Can you work these out from the model? Positions are in its coordinate system, mm. Face numbers are marked on the shaded views. A direction names the side the tool comes from. Coordinates: 2 decimals unless noted, no trailing zeros. Loops run counter-clockwise (first coordinate to the right, second up) from the corner with the lowest first, then second, coordinate; pieces in that order, holes last. Notation, with made-up numbers: M 3.5,22.5 L 27.5,22.5 A21 ccw 27.5,42.5 Z; hole C 34.25,20 d1. An arc over 180 degrees is marked long. Return JSON: item names as keys, results as strings. Group by question number.
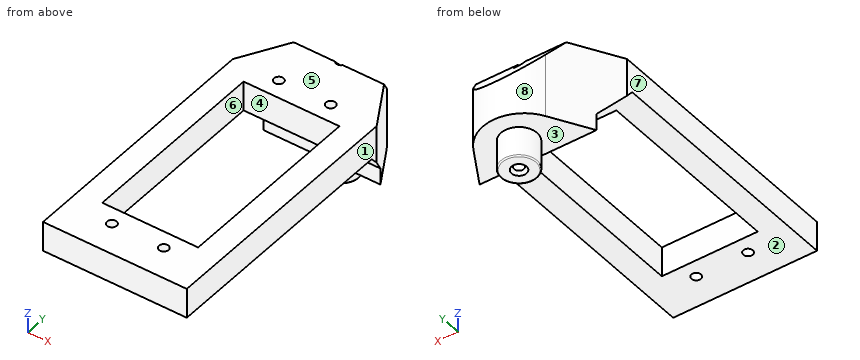
```python
from build123d import *

# Parameters (mm, degrees)
F0_R           = 1.016
F0_W           = 20.32
F0_H           = 40.64
F2_DEPTH       = 17.526
F3_START       = -25.4
F3_DEPTH       = 40.641
F4_R           = 3.81
F5_DEPTH       = 6.35
F7_D           = 2.032
F7_CSINK_D     = 3.175
F7_CSINK_ANGLE = 82
F8_R           = 0.254


with BuildPart() as f2:
    # F0 (on Top) → F2 (new body, through all)
    with BuildSketch(Plane.XY):
        with BuildLine():
            Line((-15.24, -40.64), (15.24, -40.64))
            Line((15.24, -40.64), (15.24, 13.97))
            Line((15.24, 13.97), (7.62, 27.1682271537))
            ThreePointArc((7.62, 27.1682271537), (0, 31.6135833353), (-7.62, 27.1682271537))
            Line((-7.62, 27.1682271537), (-15.24, 13.97))
            Line((-15.24, 13.97), (-15.24, -40.64))
        make_face()
        with Locations((-5.4991, -34.036)):
            Circle(F0_R, mode=Mode.SUBTRACT)
        with Locations((5.4991, -34.036)):
            Circle(F0_R, mode=Mode.SUBTRACT)
        with Locations((0, -10.16)):
            Rectangle(F0_W, F0_H, mode=Mode.SUBTRACT)
        with Locations((-5.4991, 13.97)):
            Circle(F0_R, mode=Mode.SUBTRACT)
        with Locations((5.4991, 13.97)):
            Circle(F0_R, mode=Mode.SUBTRACT)
    extrude(amount=F2_DEPTH)

    # F1 (on Right) → F3 (intersect)
    with BuildSketch(Plane.YZ.offset(F3_START)):
        Polygon((18.9135833353, 3.556), (18.9135833353, 0), (31.6135833353, 0), (31.6135833353, 8.1784219752), (23.7700340623, 17.526), (-40.64, 17.526), (-40.64, 11.176), (12.5196441457, 11.176), align=None)
    extrude(amount=F3_DEPTH, mode=Mode.INTERSECT)

    # F4 (on face) → F5 (join)
    with BuildSketch(Plane.XY):
        with Locations((0, 24.3734540549)):
            Circle(F4_R)
    extrude(amount=-F5_DEPTH)

    # F7 (through all)
    with Locations(Plane(origin=(0, 0, -6.35), x_dir=(1, 0, 0), z_dir=(0, 0, -1))):
        with Locations((0, -24.3734540549)):
            CounterSinkHole(F7_D / 2, F7_CSINK_D / 2, counter_sink_angle=F7_CSINK_ANGLE)

    # F8
    f8_edges = [f2.edges().sort_by_distance(p)[0] for p in [
        (-3.81, 24.373454, -6.35),
    ]]
    fillet(f8_edges, radius=F8_R)


solid = f2.part
```
1) Suppose I cut it at D-D, the plane x = -11.5. List the corners of the cut face in (y, z) for me, then the cut area to 3 significant figures.
2) For pin 1 (4 mm diameter, centred on x = -5, z = 2, fed in from -Y); pin 2 (3.5 mm diameter, centred on x = -5.5, y = 13.97, fed in from -Z); pin 3 (2.5 mm diameter, centred on x = 5.5, y = -34.04, fed in from -Z); pin 4 (2.5 mm diameter, centred on x = 5.5, y = 13.97, fed in from +Z), each with a flat end and sliding along its axis, tell me the tip position at first contact or that it passes through.
3) Suppose I cut it at B-B, the plane x = 0. List the corners of the cut face in (y, z) for me.
4) If I drill on line 1 (X direction, y = 13.97, z = 15.75); line 2 (Y direction, x = 0, z = 2.5); line 3 (Y direction, x = 14.5, z = 16), over which ranges is the centre line in solid material (lowest first)? Write a range as from..to.
5) For the marked faces 1, 2, 3, 4 and 5, which set-ups out of +Z, -Z, +X, -X, +Y, -Y let a thin tool reach every point of the face, with its end or its side?
6) If we mould it in two halves opening along Y, with no side actions, what happens to the marked faces 6, 7 and 8? For each: +Y half, -Y half, draft (parallel to the pull), parting line (faces both ways), or undercut.
7) Suppose I cut it at C-C, the plane z = 2.25. List the corners of the cut face in (x, y) for me.
8) Suppose I cut it at A-A, the plane y = -14. List the corners of the cut face in (x, z) for me, then the cut area to 3 significant figures.
Returned:
{
 "1": {"outline": "M -40.64,11.18 L 12.52,11.18 L 18.91,3.56 L 18.91,0 L 20.45,0 L 20.45,17.53 L -40.64,17.53 Z", "area": "429 mm²"},
 "2": {"pin 1": "stops at y = 18.54", "pin 2": "stops at z = 7.36", "pin 3": "stops at z = 11.18", "pin 4": "stops at z = 17.53"},
 "3": {"outline": "M -40.64,11.18 L -30.48,11.18 L -30.48,17.53 L -40.64,17.53 Z; M 10.16,11.18 L 12.52,11.18 L 18.91,3.56 L 18.91,0 L 20.56,0 L 20.56,-6.1 A0.25 ccw 20.82,-6.35 L 22.79,-6.35 L 23.36,-5.69 L 23.36,17.53 L 10.16,17.53 Z; M 25.39,-5.69 L 25.96,-6.35 L 27.93,-6.35 A0.25 ccw 28.18,-6.1 L 28.18,0 L 31.61,0 L 31.61,8.18 L 25.39,15.6 Z"},
 "4": {"line 1": "x = -15.24..-6.52, -4.48..4.48, 6.52..15.24", "line 2": "y = 18.91..23.36, 25.39..31.61", "line 3": "y = -40.64..15.25"},
 "5": {"face 1": "+Z, -Z, +X, +Y, -Y", "face 2": "-Z, +X, -X, -Y", "face 3": "-Z", "face 4": "+Z, -Z", "face 5": "+Z, +X, -X, +Y, -Y"},
 "6": {"face 6": "undercut", "face 7": "draft", "face 8": "+Y half"},
 "7": {"outline": "M -12.39,18.91 L 12.39,18.91 L 7.62,27.17 A8.75 ccw -7.62,27.17 Z; hole C 0,24.37 d2.03"},
 "8": {"outline": "M -15.24,11.18 L -10.16,11.18 L -10.16,17.53 L -15.24,17.53 Z; M 10.16,11.18 L 15.24,11.18 L 15.24,17.53 L 10.16,17.53 Z", "area": "64.5 mm²"}
}
